Work out the finished part from the listing and answer in its coordinate system (mm). A direction names the side the tool comes from. Coordinates: 2 decimals unless noted, no trailing zeros. Order: outer loops, then holes, each group sorted by start corner. A loop starts at its lowest first (then second) coordinate and runs counter-clockwise, first axis right, second up. Notation, with made-up numbers: (34.5, -39) -> (75.5, -39) arc R9 cw to (75.5, -30) -> close; hole circle Ø1 at (22.5, 57). An arc over 180 degrees is marked (long way). Answer as CSV lines item,"result". Start each with the question number.
Item 1: Section D-D (y = -42) is taken. Write down the section's boundary in (x, z).
Item 2: For a pull along X with two mould halves and no side action, classify faces 3 (the face through (48.21, -27.65, 6.26)), 4 (the face through (-53.5, -24.9, 12.7)), 5 (the face through (20.763, -25.481, 16.322)) as pulls with the +X half, pulls with the -X half, needs draft (parallel to the pull), parting line crosses it, or undercut.
Item 3: Section C-C (z = 33.5) is taken. Write down the section's boundary in (x, y).
Item 4: Section A-A (y = -22) is taken. Write down the section's boundary in (x, z).
Item 5: Straight lines are drawn through the part: L1, parallel to X at y = -28, z = 25; L2, parallel to Z at x = 55, y = -9.5; L3, parallel to X at y = -32, z = 23. For each, find the intervals that lie inside material, in ascending order.
Item 6: Section B-B (x = -48) is taken. Write down the section's boundary in (y, z).
Item 7: Each of these flat-tipped pins is pushed along its axis until it touches: pin 1 Ø12 at (y, z) = (-11, 38) entering from -X; pin 2 Ø6 at (x, y) = (47, -12.5) entering from +Z; pin 3 Ø5 at (x, y) = (-12, -12) entering from +Z. Where does it stop, or does it pass through?
Item 8: Which of the six approach directions +Z, -Z, +X, -X, +Y, -Y give full straight-line access (tool end or side, diameter ignored) to faces 1 (the face through (-65.606, -25, 6)), 2 (the face through (49, -25, 12.7))?
```python
from build123d import *

# Parameters (mm, degrees)
F0_W     = 127
F0_H     = 38.1
F0_R     = 6.35
F1_DEPTH = 12.7
F3_DEPTH = 38.1


with BuildPart() as f1:
    # F0 (on Top) → F1 (new body)
    with BuildSketch(Plane.XY):
        with Locations((-2.1062232554, -25.2138755785)):
            Rectangle(F0_W, F0_H)
        with Locations((-46.5562232554, -25.2138755785)):
            Circle(F0_R, mode=Mode.SUBTRACT)
        with Locations((42.3437767446, -25.2138755785)):
            Circle(F0_R, mode=Mode.SUBTRACT)
    extrude(amount=F1_DEPTH)

    # F2 (on face) → F3 (join, through all)
    with BuildSketch(Plane.XZ.offset(44.2638755785)):
        with BuildLine():
            ThreePointArc((12.0928084017, 12.7), (15.6897601828, 18.6025391898), (16.9437767446, 25.4))
            ThreePointArc((16.9437767446, 25.4), (-2.1062232554, 44.45), (-21.1562232554, 25.4))
            ThreePointArc((-21.1562232554, 25.4), (-19.9022066936, 18.6025391898), (-16.3052549125, 12.7))
            Line((-16.3052549125, 12.7), (-2.1062232095, 12.7))
            Line((-2.1062232095, 12.7), (12.0928084017, 12.7))
        make_face()
        with BuildLine():
            ThreePointArc((10.5937767446, 25.4), (6.8740328819, 16.4197438952), (-2.1062232095, 12.7))
            ThreePointArc((-2.1062232095, 12.7), (-11.0864793927, 34.3802561048), (10.5937767446, 25.4))
        make_face(mode=Mode.SUBTRACT)
        with BuildLine():
            ThreePointArc((29.6437767446, 12.7), (20.6635206235, 16.4197438789), (16.9437767446, 25.4))
            ThreePointArc((16.9437767446, 25.4), (15.6897601828, 18.6025391898), (12.0928084017, 12.7))
            Line((12.0928084017, 12.7), (29.6437767446, 12.7))
        make_face()
        with BuildLine():
            ThreePointArc((-16.3052549125, 12.7), (-19.9022066936, 18.6025391898), (-21.1562232554, 25.4))
            ThreePointArc((-21.1562232554, 25.4), (-24.8759671343, 16.4197438789), (-33.8562232554, 12.7))
            Line((-33.8562232554, 12.7), (-16.3052549125, 12.7))
        make_face()
        with BuildLine():
            ThreePointArc((-16.3052549125, 12.7), (-2.1062232554, 6.35), (12.0928084017, 12.7))
            Line((12.0928084017, 12.7), (-2.1062232095, 12.7))
            Line((-2.1062232095, 12.7), (-16.3052549125, 12.7))
        make_face()
    extrude(amount=-F3_DEPTH)


solid = f1.part
```
Checked values:
1,outline,"(-65.61, 0) -> (61.39, 0) -> (61.39, 12.7) -> (29.64, 12.7) arc R12.7 cw to (16.94, 25.4) arc R19.05 ccw to (-21.16, 25.4) arc R12.7 cw to (-33.86, 12.7) -> (-65.61, 12.7) -> close; hole circle Ø25.4 at (-2.11, 25.4)"
2,face 3,"undercut"
2,face 4,"needs draft"
2,face 5,"pulls with the +X half"
3,outline,"(-19.35, -44.26) -> (-11.89, -44.26) -> (-11.89, -6.16) -> (-19.35, -6.16) -> close; (7.68, -44.26) -> (15.14, -44.26) -> (15.14, -6.16) -> (7.68, -6.16) -> close"
4,outline,"(-65.61, 0) -> (-52.03, 0) -> (-52.03, 12.7) -> (-65.61, 12.7) -> close; (-41.08, 0) -> (36.87, 0) -> (36.87, 12.7) -> (29.64, 12.7) arc R12.7 cw to (16.94, 25.4) arc R19.05 ccw to (-21.16, 25.4) arc R12.7 cw to (-33.86, 12.7) -> (-41.08, 12.7) -> close; (47.82, 0) -> (61.39, 0) -> (61.39, 12.7) -> (47.82, 12.7) -> close; hole circle Ø25.4 at (-2.11, 25.4)"
5,L1,"x = -21.16 to -14.8, 10.59 to 16.95"
5,L2,"z = 0 to 12.7"
5,L3,"x = -21.39 to -14.58, 10.36 to 17.17"
6,outline,"(-44.26, 0) -> (-31.4, 0) -> (-31.4, 12.7) -> (-44.26, 12.7) -> close; (-19.03, 0) -> (-6.16, 0) -> (-6.16, 12.7) -> (-19.03, 12.7) -> close"
7,pin 1,"stops at x = -19.98"
7,pin 2,"stops at z = 12.7"
7,pin 3,"stops at z = 42.96"
8,face 1,"+Z, -Z, -X, +Y, -Y"
8,face 2,"+Z, +X, +Y, -Y"
